Geometry check sheet. Reference: the model listing, model coordinates, mm. Round coordinates to 2 decimals unless told otherwise and drop trailing zeros. Order: outer loops, then holes, each group sorted by start corner. A loop starts at its lowest first (then second) coordinate and runs counter-clockwise, first axis right, second up.
```python
from build123d import *

# Parameters (mm, degrees)
F0_W         = 69.85
F0_H         = 101.6
F1_DEPTH     = 6.35
F2_R         = 5.08
F3_T1_DEPTH  = 13.97
F3_S5_W      = 5.08
F3_S5_H      = 5.08
F3_T6_DEPTH  = 5.08
F3_S11_W     = 5.08
F3_S11_H     = 5.08
F3_T12_DEPTH = 5.08
F3_S17_W     = 5.08
F3_S17_H     = 5.08
F3_T18_DEPTH = 5.08
F3_S23_W     = 5.08
F3_S23_H     = 5.08
F3_T24_DEPTH = 5.08


# Not quite as in the source:
# - a fillet or chamfer that OpenCascade refuses, or shapes differently, is made with other operations: its cross-section is extruded or revolved along the edge and cut away or added


with BuildPart() as f1:
    # F0 (on Top) → F1 (new body)
    with BuildSketch(Plane.XY):
        with Locations((34.925, -50.8)):
            Rectangle(F0_W, F0_H)
    extrude(amount=F1_DEPTH)

    # F2
    f2_edges = [f1.edges().sort_by_distance(p)[0] for p in [
        (69.85, -50.8, 0),
        (34.925, -101.6, 0),
        (0, -50.8, 0),
        (34.925, 0, 0),
    ]]
    fillet(f2_edges, radius=F2_R)

    # F3: fillet of radius 5.08 on 4 edges, made by hand

    # F3_s2 → F3_t1 (cut)
    with BuildSketch(Plane.XY.offset(5.08)):
        with BuildLine():
            ThreePointArc((0, -96.52), (1.4878975516, -100.1121024484), (5.08, -101.6))
            Line((5.08, -101.6), (0, -101.6))
            Line((0, -101.6), (0, -96.52))
        make_face()
        with BuildLine():
            ThreePointArc((64.77, 0), (68.3621024484, -1.4878975516), (69.85, -5.08))
            Line((69.85, -5.08), (69.85, 0))
            Line((69.85, 0), (64.77, 0))
        make_face()
        with BuildLine():
            ThreePointArc((5.08, 0), (1.4878975516, -1.4878975516), (0, -5.08))
            Line((0, -5.08), (0, 0))
            Line((0, 0), (5.08, 0))
        make_face()
        with BuildLine():
            ThreePointArc((69.85, -96.52), (68.3621024484, -100.1121024484), (64.77, -101.6))
            Line((64.77, -101.6), (69.85, -101.6))
            Line((69.85, -101.6), (69.85, -96.52))
        make_face()
    extrude(amount=F3_T1_DEPTH, mode=Mode.SUBTRACT)


with BuildPart() as f3_tool4:
    # F3_s5 → F3_t6 (new body)
    with BuildSketch(Plane.YZ.offset(64.77)):
        with Locations((-99.06, 2.54)):
            Rectangle(F3_S5_W, F3_S5_H)
    extrude(amount=F3_T6_DEPTH)

    # F3_s7 → F3_t8 (revolve, cut)
    with BuildSketch(Plane(origin=(64.77, -96.52, 5.08), x_dir=(0, 0.7071067812, 0.7071067812), z_dir=(0, 0.7071067812, -0.7071067812))):
        with BuildLine():
            ThreePointArc((0, -5.08), (5.08, 0), (0, 5.08))
            Line((0, 5.08), (0, -5.08))
        make_face()
    revolve(axis=Axis((64.77, -96.52, 5.08), (1, 0, 0)), mode=Mode.SUBTRACT)


with BuildPart() as f1_1:
    add(f1.part)

    # F3_t3: cut F3_tool4
    add(f3_tool4.part, mode=Mode.SUBTRACT)


with BuildPart() as f3_tool10:
    # F3_s11 → F3_t12 (new body)
    with BuildSketch(Plane.XZ.offset(5.08)):
        with Locations((2.54, 2.54)):
            Rectangle(F3_S11_W, F3_S11_H)
    extrude(amount=-F3_T12_DEPTH)

    # F3_s13 → F3_t14 (revolve, cut)
    with BuildSketch(Plane(origin=(5.08, -5.08, 5.08), x_dir=(0.7071067812, 0, 0.7071067812), z_dir=(-0.7071067812, 0, 0.7071067812))):
        with BuildLine():
            ThreePointArc((0, -5.08), (5.08, 0), (0, 5.08))
            Line((0, 5.08), (0, -5.08))
        make_face()
    revolve(axis=Axis((5.08, -5.08, 5.08), (0, 1, 0)), mode=Mode.SUBTRACT)


with BuildPart() as f1_2:
    add(f1_1.part)

    # F3_t9: cut F3_tool10
    add(f3_tool10.part, mode=Mode.SUBTRACT)


with BuildPart() as f3_tool16:
    # F3_s17 → F3_t18 (new body)
    with BuildSketch(Plane.XZ.offset(5.08)):
        with Locations((67.31, 2.54)):
            Rectangle(F3_S17_W, F3_S17_H)
    extrude(amount=-F3_T18_DEPTH)

    # F3_s19 → F3_t20 (revolve, cut)
    with BuildSketch(Plane(origin=(64.77, -5.08, 5.08), x_dir=(-0.7071067812, 0, 0.7071067812), z_dir=(-0.7071067812, 0, -0.7071067812))):
        with BuildLine():
            ThreePointArc((0, -5.08), (5.08, 0), (0, 5.08))
            Line((0, 5.08), (0, -5.08))
        make_face()
    revolve(axis=Axis((64.77, -5.08, 5.08), (0, 1, 0)), mode=Mode.SUBTRACT)


with BuildPart() as f1_3:
    add(f1_2.part)

    # F3_t15: cut F3_tool16
    add(f3_tool16.part, mode=Mode.SUBTRACT)


with BuildPart() as f3_tool22:
    # F3_s23 → F3_t24 (new body)
    with BuildSketch(Plane.YZ.offset(5.08)):
        with Locations((-99.06, 2.54)):
            Rectangle(F3_S23_W, F3_S23_H)
    extrude(amount=-F3_T24_DEPTH)

    # F3_s25 → F3_t26 (revolve, cut)
    with BuildSketch(Plane(origin=(5.08, -96.52, 5.08), x_dir=(0, 0.7071067812, 0.7071067812), z_dir=(0, -0.7071067812, 0.7071067812))):
        with BuildLine():
            ThreePointArc((0, -5.08), (5.08, 0), (0, 5.08))
            Line((0, 5.08), (0, -5.08))
        make_face()
    revolve(axis=Axis((5.08, -96.52, 5.08), (-1, 0, 0)), mode=Mode.SUBTRACT)


with BuildPart() as f1_4:
    add(f1_3.part)

    # F3_t21: cut F3_tool22
    add(f3_tool22.part, mode=Mode.SUBTRACT)


solid = f1_4.part
```
(1) Material ranges on line 1 (X direction, y = -60, z = 4.75); line 2 (X direction, y = -22.5, z = 1); line 3 (Y direction, x = 28, z = 5), recorded low to high.
Returned:
line 1: x = 0.01 to 69.84
line 2: x = 2.05 to 67.8
line 3: y = -101.6 to 0
(2) Sectioned sample at C-C, the plane y = -22. Record the cut outline in (x, z).
Returned:
outline: (0, 5.08) arc R5.08 ccw to (5.08, 0) - (64.77, 0) arc R5.08 ccw to (69.85, 5.08) - (69.85, 6.35) - (0, 6.35) - close
(3) Sectioned sample at A-A, the plane x = 26. Record the cut outline in (y, z).
Returned:
outline: (-101.6, 5.08) arc R5.08 ccw to (-96.52, 0) - (-5.08, 0) arc R5.08 ccw to (0, 5.08) - (0, 6.35) - (-101.6, 6.35) - close
(4) Depth check by flat-ended pin: P1, Ø2, axis at y = -63, z = 3, coming from the -X side. Enter the tip coordinate at first touch or a pass-through.
Returned:
P1: stops at x = 0.12
(5) Sectioned sample at B-B, the plane z = 1.5. Record the cut outline in (x, y), and give its area (3 significant figures).
Returned:
outline: (1.48, -96.52) arc R3.6 ccw to (5.08, -100.12) - (64.77, -100.12) arc R3.6 ccw to (68.37, -96.52) - (68.37, -5.08) arc R3.6 ccw to (64.77, -1.48) - (5.08, -1.48) arc R3.6 ccw to (1.48, -5.08) - close
area: 6,590 mm2
